Could you check a few things on this model? Use its own coordinates, in mm. A direction names the side the tool comes from. Give positions to 0.01 mm unless a question says otherwise; leave off trailing zeros. Write each loop counter-clockwise with the first axis right and the second up, starting at its lowest first coordinate (ties: lowest second). Pieces come first, ordered by that corner, then holes. Notation, with made-up numbers: M 57,13 L 106,13 A13 cw 106,26 Z; hole C -24,46 d11. An arc over 180 degrees is marked long. One line per item, written item: value.
```python
from build123d import *

# Parameters (mm, degrees)
BOSS_EXTRUDE1_DEPTH = 5.75
CIRPATTERN1_COUNT   = 20
SKETCH2_R           = 11.945
BOSS_EXTRUDE2_DEPTH = 1.5
SKETCH4_R           = 8
CUT_EXTRUDE2_DEPTH  = 5
SKETCH3_R           = 3.2
CUT_EXTRUDE1_DEPTH  = 14.5


with BuildPart() as part:
    # Sketch1 → Boss-Extrude1 (new, symmetric)
    with BuildSketch(Plane(origin=(0, 0, 0), x_dir=(0, 0, -1), z_dir=(1, 0, 0))):
        with BuildLine():
            Line((0, 13.285), (0, 0))
            Line((0, 0), (4.10529077, 12.634785819))
            ThreePointArc((4.10529077, 12.634785819), (3.221971668, 13.384600745), (3.120582785, 14.538808418))
            ThreePointArc((3.120582785, 14.538808418), (3.07819699, 14.888914891), (2.788180956, 15.089568316))
            ThreePointArc((2.788180956, 15.089568316), (2.400486866, 15.156077586), (2.011215381, 15.212627574))
            ThreePointArc((2.011215381, 15.212627574), (1.673388423, 15.111414709), (1.524888287, 14.791541599))
            ThreePointArc((1.524888287, 14.791541599), (1.071791943, 13.725155757), (0, 13.285))
        make_face()
    boss_extrude1 = extrude(amount=BOSS_EXTRUDE1_DEPTH, both=True)

    # CirPattern1: Boss-Extrude1 ×20 about axis
    cirpattern1_axis = Axis((0, 0, 0), (1, 0, 0))
    for i in range(1, CIRPATTERN1_COUNT):
        add(boss_extrude1.rotate(cirpattern1_axis, i * 360 / CIRPATTERN1_COUNT))

    # Sketch2 → Boss-Extrude2 (add)
    with BuildSketch(Plane(origin=(5.75, 0, 0), x_dir=(0, 0, -1), z_dir=(1, 0, 0))):
        Circle(SKETCH2_R)
    boss_extrude2 = extrude(amount=BOSS_EXTRUDE2_DEPTH)

    # Sketch4 → Cut-Extrude2 (cut)
    with BuildSketch(Plane(origin=(7.25, 0, 0), x_dir=(0, 0, -1), z_dir=(1, 0, 0))):
        Circle(SKETCH4_R)
    cut_extrude2 = extrude(amount=-CUT_EXTRUDE2_DEPTH, mode=Mode.SUBTRACT)

    # Mirror1: Boss-Extrude2, Cut-Extrude2 across plane
    add(boss_extrude2.mirror(Plane(origin=(0, 0, 0), x_dir=(0, 0, 1), z_dir=(1, 0, 0))))
    add(cut_extrude2.mirror(Plane(origin=(0, 0, 0), x_dir=(0, 0, 1), z_dir=(1, 0, 0))), mode=Mode.SUBTRACT)

    # Sketch3 → Cut-Extrude1 (cut)
    with BuildSketch(Plane(origin=(7.25, 0, 0), x_dir=(0, 0, -1), z_dir=(1, 0, 0))):
        Circle(SKETCH3_R)
    extrude(amount=-CUT_EXTRUDE1_DEPTH, mode=Mode.SUBTRACT)


solid = part.part
```
1) If we section it at A-A, the plane z = -4.5: Write out the boundary of the cut face in (x, y).
Outcome:
outline: M -7.25,-11.06 L -5.75,-11.06 L -5.75,-12.56 L 5.75,-12.56 L 5.75,-11.06 L 7.25,-11.06 L 7.25,-6.61 L 2.25,-6.61 L 2.25,6.61 L 7.25,6.61 L 7.25,11.06 L 5.75,11.06 L 5.75,12.56 L -5.75,12.56 L -5.75,11.06 L -7.25,11.06 L -7.25,6.61 L -2.25,6.61 L -2.25,-6.61 L -7.25,-6.61 Z
2) On a 3-axis mill with a long thin cutter (end or side, diameter ignored), from which of +Z, -Z, +X, -X, +Y, -Y can I reach the whole of each face in a straight line? I mean faces 1 (the face through (4.78, -7.81, 1.73)), 2 (the face through (-4.78, -7.81, 1.73)), 3 (the face through (-7.25, -8, -2)). Say none if no direction works.
Outcome:
face 1: +X
face 2: -X
face 3: +Z, -Z, -X, +Y, -Y
3) If we section it at B-B, the plane y = 9.5: Write out the boundary of the cut face in (x, z).
Outcome:
outline: M -7.25,-7.24 L -5.75,-7.24 L -5.75,-10.68 L 5.75,-10.68 L 5.75,-7.24 L 7.25,-7.24 L 7.25,7.24 L 5.75,7.24 L 5.75,10.68 L -5.75,10.68 L -5.75,7.24 L -7.25,7.24 Z
4) I'm going to push flat-ended pins straight in: pin 1 (14.5 mm diameter, centred on y = 0, z = 0, fed in from -X); pin 2 (10 mm diameter, centred on y = 0, z = 0, fed in from +X); pin 3 (4 mm diameter, centred on x = 3, y = -5.5, fed in from -Z). Where does each tip first touch, or does it pass through?
Outcome:
pin 1: stops at x = -2.25
pin 2: stops at x = 2.25
pin 3: stops at z = -13.89
5) We'd pull the mould along Y, two halves only. Please class faces 4 (the face through (-2.25, 0.1, -3.4)), 5 (the face through (6.49, -7.27, 9.48)), 6 (the face through (-5.75, 10.4, 6.2)): pulls with the +Y half, pulls with the -Y half, needs draft (parallel to the pull), parting line crosses it, or undercut.
Outcome:
face 4: undercut
face 5: parting line crosses it
face 6: needs draft
6) If we section it at C-C, the plane z = 9: Write out the boundary of the cut face in (x, y), then the cut area to 3 significant figures.
Outcome:
outline: M -7.25,-7.85 L -5.75,-7.85 L -5.75,-10.49 L 5.75,-10.49 L 5.75,-7.85 L 7.25,-7.85 L 7.25,7.85 L 5.75,7.85 L 5.75,10.49 L -5.75,10.49 L -5.75,7.85 L -7.25,7.85 Z
area: 288 mm^2
7) Please list where these lines run through material, in increasing order: L1, parallel to Y at x = 2, z = 13; L2, parallel to X at y = 5.5, z = 2.5; L3, parallel to Y at x = 4, z = -5 (3 decimals). Write a range as from..to.
Outcome:
L1: y = -7.52..-5.65, -3.51..3.51, 5.65..7.52
L2: x = -2.25..2.25
L3: y = -12.62..-6.245, 6.245..12.62
